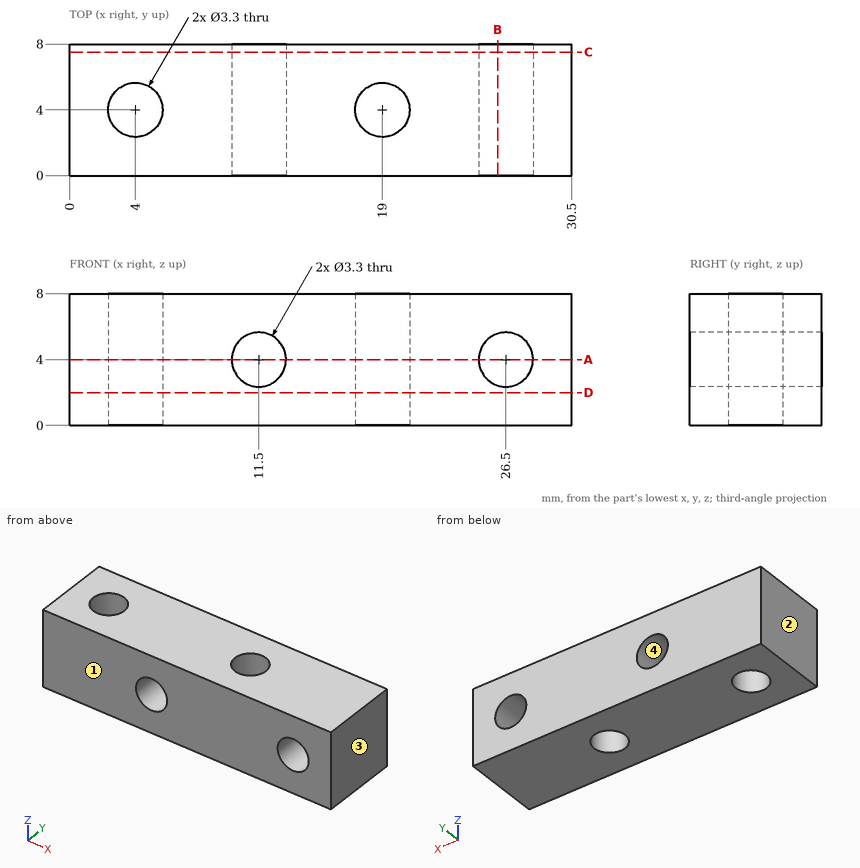
Geometry: see drawing. Coordinates: mm, zero at the bounding-box minimum. Give positions to 0.01 mm unless a question says otherwise; leave off trailing zeros. Loops run counter-clockwise (first coordinate to the right, second up) from the corner with the lowest first, then second, coordinate; pieces in that order, holes last. Notation, with made-up numbers: (69.5, 27.25) -> (91.5, 27.25) arc R11 ccw to (91.5, 47.25) -> close; hole circle Ø7 at (30, -33.5). An arc over 180 degrees is marked (long way). Answer as a JSON object with one key per item and string values. Group by question number.
Item 1: Cut plane B-B, the plane x = 26. Return the cut outline in (y, z).
Item 2: Line query: probe 1 along X at (y, z) = (0.75, 4); probe 2 along X at (y, z) = (5.25, 4); probe 3 along X at (y, z) = (0.75, 3.25). Output: solid intervals per line, ascending.
Item 3: Cut plane D-D, the plane z = 2. Return the cut outline in (x, y).
Item 4: Cut plane C-C, the plane y = 7.5. Return the cut outline in (x, z), and give its area (3 significant figures).
Item 5: Cut plane A-A, the plane z = 4. Return the cut outline in (x, y).
Item 6: Pull-direction query (X, two-part tool) for the marked faces 1, 2, 3 and 4; classes: released by +X, released by -X, zero draft, split by the parting line, or undercut.
Checks:
{
 "1": {"outline": "(0, 0) -> (8, 0) -> (8, 2.43) -> (0, 2.43) -> close; (0, 5.57) -> (8, 5.57) -> (8, 8) -> (0, 8) -> close"},
 "2": {"probe 1": "x = 0 to 9.85, 13.15 to 24.85, 28.15 to 30.5", "probe 2": "x = 0 to 2.92, 5.08 to 9.85, 13.15 to 17.92, 20.08 to 24.85, 28.15 to 30.5", "probe 3": "x = 0 to 10.03, 12.97 to 25.03, 27.97 to 30.5"},
 "3": {"outline": "(0, 0) -> (30.5, 0) -> (30.5, 8) -> (0, 8) -> close; hole circle Ø3.3 at (4, 4); hole circle Ø3.3 at (19, 4)"},
 "4": {"outline": "(0, 0) -> (30.5, 0) -> (30.5, 8) -> (0, 8) -> close; hole circle Ø3.3 at (11.5, 4); hole circle Ø3.3 at (26.5, 4)", "area": "227 mm²"},
 "5": {"outline": "(0, 0) -> (9.85, 0) -> (9.85, 8) -> (0, 8) -> close; (13.15, 0) -> (24.85, 0) -> (24.85, 8) -> (13.15, 8) -> close; (28.15, 0) -> (30.5, 0) -> (30.5, 8) -> (28.15, 8) -> close; hole circle Ø3.3 at (4, 4); hole circle Ø3.3 at (19, 4)"},
 "6": {"face 1": "zero draft", "face 2": "released by -X", "face 3": "released by +X", "face 4": "undercut"}
}
